Geometry: see drawing. Coordinates: mm, zero at the bounding-box minimum. A direction names the side the tool comes from. Coordinates: 2 decimals unless noted, no trailing zeros. Loops run counter-clockwise (first coordinate to the right, second up) from the corner with the lowest first, then second, coordinate; pieces in that order, holes last. Notation, with made-up numbers: (-30, -24.5) -> (-4, -24.5) arc R15 ccw to (-4, 4.5) -> close; hole circle Ø8 at (64, 7). An arc over 180 degrees is marked (long way). Answer as a JSON object with one key per item and string values.
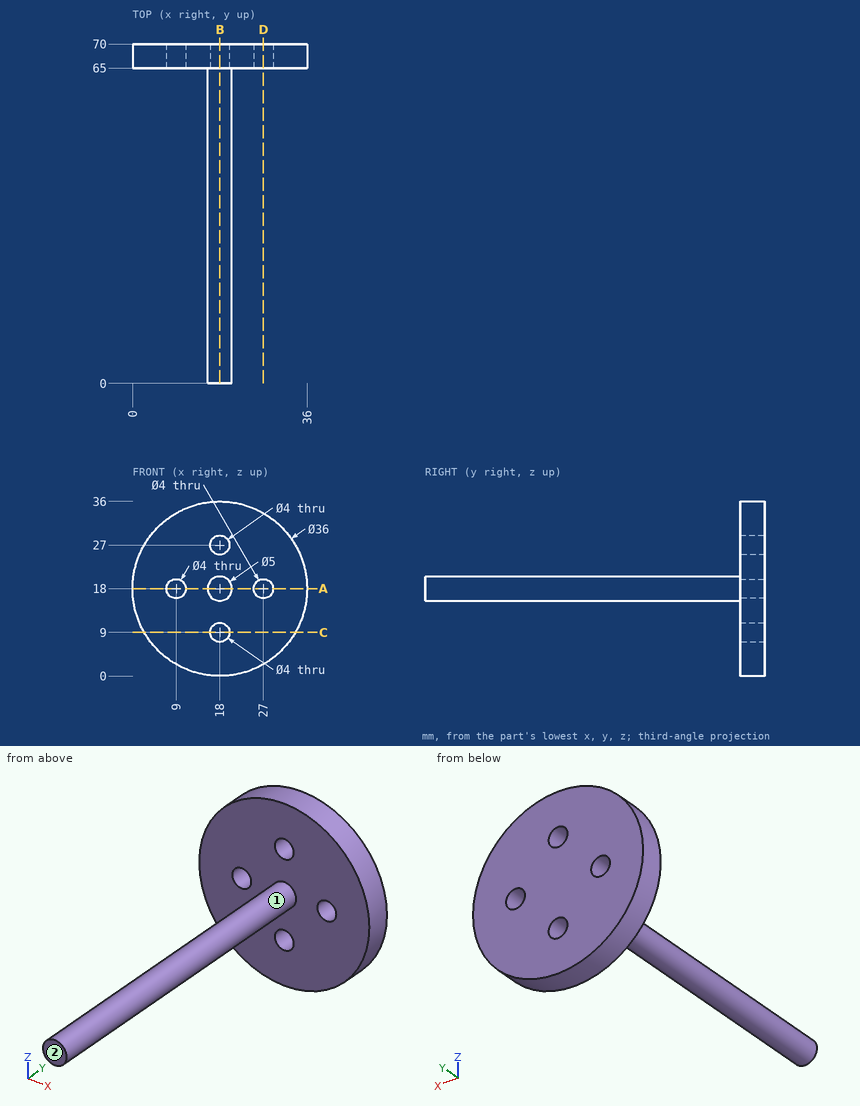
1. Section query D-D (x = 27). Return loops of the section in (y, z), plus the area to 3 significant figures.
Reply:
{"outline": "(65, 2.41) -> (70, 2.41) -> (70, 16) -> (65, 16) -> close; (65, 20) -> (70, 20) -> (70, 33.59) -> (65, 33.59) -> close", "area": "136 mm2"}
2. Line query: line 1 along X through (y, z) = (68.25, 18); line 2 along Y through (x, z) = (27, 14.5); line 3 along X through (y, z) = (66, 9). Output: solid intervals per line, ascending.
Reply:
{"line 1": "x = 0 to 7, 11 to 25, 29 to 36", "line 2": "y = 65 to 70", "line 3": "x = 2.41 to 16, 20 to 33.59"}
3. Section query C-C (z = 9). Return loops of the section in (x, y), plus the area to 3 significant figures.
Reply:
{"outline": "(2.41, 65) -> (16, 65) -> (16, 70) -> (2.41, 70) -> close; (20, 65) -> (33.59, 65) -> (33.59, 70) -> (20, 70) -> close", "area": "136 mm2"}
4. Access query for the marked faces 1 and 2. Directions: +Z, -Z, +X, -X, +Y, -Y. A direction counts if a zero-diameter tool reaches every point of the face in a straight line with its end or side. Return the directions, or none.
Reply:
{"face 1": "-Y", "face 2": "+Z, -Z, +X, -X, -Y"}
5. Section query A-A (z = 18). Return loops of the section in (x, y).
Reply:
{"outline": "(0, 65) -> (7, 65) -> (7, 70) -> (0, 70) -> close; (11, 65) -> (15.5, 65) -> (15.5, 0) -> (20.5, 0) -> (20.5, 65) -> (25, 65) -> (25, 70) -> (11, 70) -> close; (29, 65) -> (36, 65) -> (36, 70) -> (29, 70) -> close"}
6. Section query B-B (x = 18). Return loops of the section in (y, z).
Reply:
{"outline": "(0, 15.5) -> (65, 15.5) -> (65, 11) -> (70, 11) -> (70, 25) -> (65, 25) -> (65, 20.5) -> (0, 20.5) -> close; (65, 0) -> (70, 0) -> (70, 7) -> (65, 7) -> close; (65, 29) -> (70, 29) -> (70, 36) -> (65, 36) -> close"}
7. Pin query (flat end, axial travel): P1, Ø6.5, axis at x = 9, z = 18, coming from the -Y side; P2, Ø6.5, axis at x = 18, z = 9, coming from the +Y side; P3, Ø4, axis at y = 47.5, z = 15.5, coming from the -X side. Return the tip coordinate at first contact, or that it passes through.
Reply:
{"P1": "stops at y = 65", "P2": "stops at y = 70", "P3": "stops at x = 15.55"}
